Could you check a few things on this model? Use its own coordinates, in mm. A direction names the side the tool comes from. Coordinates: 2 decimals unless noted, no trailing zeros. Order: outer loops, then holes, each group sorted by start corner. A loop starts at its lowest first (then second) coordinate and runs counter-clockwise, first axis right, second up. Notation, with made-up numbers: (-37.75, 5) -> (18.25, 5) arc R26 cw to (18.25, 35) -> close; hole circle Ø5 at (48, -33.5). An arc over 180 degrees is marked (long way). Put each result on its own line as item: value. Start each with the question number.
Q1. Please list where these lines run through material, in increasing order: line 1 along X through (y, z) = (9, 3.3); line 2 along Y through (x, z) = (18.4, 2); line 3 along X through (y, z) = (12.5, 3.7).
Q2. We'd pull the mould along X, two halves only. Please class faces 3 (the face through (22.8, -43.6, 2)), 4 (the face through (-10.83, -32.023, 1.972)), 5 (the face through (5, -13, 0)): +X half, -X half, draft (parallel to the pull), parting line (faces both ways), or undercut.
Q3. If we section it at B-B (x = -1): Please give me the cut outline in (y, z).
Q4. If we section it at C-C (y = -22): Please give me the cut outline in (x, z), and give its area (3 significant figures).
Q5. If we section it at D-D (z = 2.35): Count the separate pieces of the cut face and the enclosed holes in it, and give its area (3 significant figures).
Q6. If we section it at A-A (y = -1.5): Please give me the cut outline in (x, z), and give its area (3 significant figures).
Q7. Will these pins go through, and if not, where does the flat tip stop? pin 1 (8 mm diameter, centred on x = -1.5, y = -22.5, fed in from -Z); pin 2 (2 mm diameter, centred on y = -46.5, z = 2, fed in from +X); pin 3 (0.9 mm diameter, centred on y = -42, z = 2.5, fed in from -X).
Q8. For faces 1 (the face through (2.77, -9.65, 1.97)), 2 (the face through (24.544, 23.862, 2.028)), which set-ups out of +Z, -Z, +X, -X, +Y, -Y let a thin tool reach every point of the face, with its end or its side?
from build123d import *

# Parameters (mm, degrees)
CROQUIS1_W              = 40
CROQUIS1_H              = 75
CROQUIS1_R              = 1.25
SALIENTE_EXTRUIR1_DEPTH = 4
CORTAR_EXTRUIR1_DEPTH   = 4
CORTAR_EXTRUIR2_DEPTH   = 4
CROQUIS4_R              = 1.6
CORTAR_EXTRUIR3_DEPTH   = 4
REDONDEO2_R             = 1.6


with BuildPart() as part:
    # Croquis1 → Saliente-Extruir1 (new body)
    with BuildSketch(Plane.XY):
        with Locations((5, -13.156453444)):
            Rectangle(CROQUIS1_W, CROQUIS1_H)
        with Locations((-8.4, -48.656453444)):
            Circle(CROQUIS1_R, mode=Mode.SUBTRACT)
        with Locations(Location((18.4, -48.656453444, 0), (0, 0, 180))):
            Circle(CROQUIS1_R, mode=Mode.SUBTRACT)
    extrude(amount=SALIENTE_EXTRUIR1_DEPTH)

    # Croquis2 → Cortar-Extruir1 (cut)
    with BuildSketch(Plane.XY.offset(4)):
        Polygon((-12, -36.656453444), (3, -9.656453444), (-12, 17.343546556), align=None)
        Polygon((-8, -40.656453444), (5, -17.256453444), (18, -40.656453444), align=None)
        Polygon((18, 21.343546556), (5, -2.056453444), (-8, 21.343546556), align=None)
        Polygon((22, 17.343546556), (7, -9.656453444), (22, -36.656453444), align=None)
    extrude(amount=-CORTAR_EXTRUIR1_DEPTH, mode=Mode.SUBTRACT)

    # Croquis3 → Cortar-Extruir2 (cut)
    with BuildSketch(Plane.XY.offset(4)):
        Polygon((-13.4, -50.656453444), (-15, -50.656453444), (-15, -40.656453444), (-15, -39.056453444), (-13.4, -40.656453444), align=None)
        Polygon((25, -50.656453444), (25, -40.656453444), (25, -39.056453444), (23.4, -40.656453444), (23.4, -50.656453444), align=None)
    extrude(amount=-CORTAR_EXTRUIR2_DEPTH, mode=Mode.SUBTRACT)

    # Croquis4 → Cortar-Extruir3 (cut)
    with BuildSketch(Plane.XY.offset(4)):
        with Locations((-14.4, -43.656453444)):
            Circle(CROQUIS4_R)
        with Locations((24.4, -43.656453444)):
            Circle(CROQUIS4_R)
    extrude(amount=-CORTAR_EXTRUIR3_DEPTH, mode=Mode.SUBTRACT)

    # Redondeo2
    redondeo2_edges = [part.edges().sort_by_distance(p)[0] for p in [
        (18, -40.656453444, 2),
        (-8, -40.656453444, 2),
        (5, -17.256453444, 2),
        (-8, 21.343546556, 2),
        (18, 21.343546556, 2),
        (5, -2.056453444, 2),
        (22, 17.343546556, 2),
        (22, -36.656453444, 2),
        (7, -9.656453444, 2),
        (-12, -36.656453444, 2),
        (-12, 17.343546556, 2),
        (3, -9.656453444, 2),
        (-15, 24.343546556, 2),
        (25, 24.343546556, 2),
        (-13.4, -40.656453444, 2),
        (-13.4, -50.656453444, 2),
        (-15, -39.056453444, 2),
        (23.4, -50.656453444, 2),
        (23.4, -40.656453444, 2),
        (25, -39.056453444, 2),
    ]]
    fillet(redondeo2_edges, radius=REDONDEO2_R)


solid = part.part
The answers:
1. line 1: -15 to -12, -7.36 to -1.14, 11.14 to 17.36, 22 to 25
1. line 2: -50.66 to -49.91, -47.41 to -30.18, 10.86 to 24.34
1. line 3: -15 to -11.29, -9.51 to -3.09, 13.09 to 19.51, 21.29 to 25
2. face 3: +X half
2. face 4: undercut
2. face 5: draft
3. outline: (-50.66, 0) -> (-40.66, 0) -> (-40.66, 4) -> (-50.66, 4) -> close; (-28.06, 0) -> (-16.86, 0) -> (-16.86, 4) -> (-28.06, 4) -> close; (-2.46, 0) -> (8.74, 0) -> (8.74, 4) -> (-2.46, 4) -> close; (21.34, 0) -> (24.34, 0) -> (24.34, 4) -> (21.34, 4) -> close
4. outline: (-15, 0) -> (-12, 0) -> (-12, 4) -> (-15, 4) -> close; (-3.86, 0) -> (2.36, 0) -> (2.36, 4) -> (-3.86, 4) -> close; (7.64, 0) -> (13.86, 0) -> (13.86, 4) -> (7.64, 4) -> close; (22, 0) -> (25, 0) -> (25, 4) -> (22, 4) -> close
4. area: 73.8 mm^2
5. separate pieces: 1
5. enclosed holes: 6
5. area: 1,570 mm^2
6. outline: (-15, 0) -> (-12, 0) -> (-12, 4) -> (-15, 4) -> close; (-1.53, 0) -> (11.53, 0) -> (11.53, 4) -> (-1.53, 4) -> close; (22, 0) -> (25, 0) -> (25, 4) -> (22, 4) -> close
6. area: 76.3 mm^2
7. pin 1: z = 0
7. pin 2: x = 23.4
7. pin 3: x = -13.4
8. face 1: +Z, -Z
8. face 2: +Z, -Z, +X, +Y
